Source: CAD feature listing. Evaluate the final solid. Frame: model axes, mm. Give positions to 0.01 mm unless a question says otherwise; leave off trailing zeros. Order: outer loops, then holes, each group sorted by start corner. A loop starts at its lowest first (then second) coordinate and runs counter-clockwise, first axis right, second up. Notation, with made-up numbers: (42, 19.5) - (46, 19.5) arc R21 ccw to (46, 34.5) - close; hole circle Ø6 at (59, 34.25). An arc over 180 degrees is marked (long way). Answer as CSV lines item,"result".
```python
from build123d import *

# Parameters (mm, degrees)
F0_R     = 12.7
F0_R_2   = 10.210562
F1_DEPTH = 1706.88
F2_R     = 6.35
F3_DEPTH = 25.4


with BuildPart() as f1:
    # F0 (on Right) → F1 (new body)
    with BuildSketch(Plane.YZ):
        Circle(F0_R)
        Circle(F0_R_2, mode=Mode.SUBTRACT)
    extrude(amount=F1_DEPTH)

    # F2 (on Top) → F3 (cut)
    with BuildSketch(Plane.XY):
        with Locations((341.376, 0)):
            Circle(F2_R)
        with Locations((682.752, 0)):
            Circle(F2_R)
        with Locations((1024.128, 0)):
            Circle(F2_R)
        with Locations((1365.504, 0)):
            Circle(F2_R)
    extrude(amount=F3_DEPTH, mode=Mode.SUBTRACT)


solid = f1.part
```
(1) Cut plane A-A (z = 0). Return loops of the section in (x, y), then the cut area to 3 significant figures.
Completed:
outline,"(0, -12.7) - (1706.88, -12.7) - (1706.88, -10.21) - (0, -10.21) - close; (0, 10.21) - (1706.88, 10.21) - (1706.88, 12.7) - (0, 12.7) - close"
area,"8,500 mm²"
(2) Cut plane B-B (y = 0). Return loops of the section in (x, z), then the cut area to 3 significant figures.
Completed:
outline,"(0, -12.7) - (1706.88, -12.7) - (1706.88, -10.21) - (0, -10.21) - close; (0, 10.21) - (335.03, 10.21) - (335.03, 12.7) - (0, 12.7) - close; (347.73, 10.21) - (676.4, 10.21) - (676.4, 12.7) - (347.73, 12.7) - close; (689.1, 10.21) - (1017.78, 10.21) - (1017.78, 12.7) - (689.1, 12.7) - close; (1030.48, 10.21) - (1359.15, 10.21) - (1359.15, 12.7) - (1030.48, 12.7) - close; (1371.85, 10.21) - (1706.88, 10.21) - (1706.88, 12.7) - (1371.85, 12.7) - close"
area,"8,370 mm²"
(3) Ray query, line 1 (X direction, y = 0, z = 11); line 2 (Z direction, x = 464.5, y = 7.75); line 3 (X direction, y = 2.5, z = 11). Return the intervals inside material, ascending. Write a range as from..to.
Completed:
line 1,"0..335.03, 347.73..676.4, 689.1..1017.78, 1030.48..1359.15, 1371.85..1706.88"
line 2,"-10.06..-6.65, 6.65..10.06"
line 3,"0..335.54, 347.21..676.91, 688.59..1018.29, 1029.97..1359.67, 1371.34..1706.88"
(4) Cut plane C-C (x = 1233). Return loops of the section in (y, z).
Completed:
outline,"circle Ø25.4 at (0, 0); hole circle Ø20.42 at (0, 0)"
(5) Contact query for flat-ended pins moving along their axis: pin 1 (2 mm diameter, centred on y = 6, z = -6.5, fed in from -X); pin 2 (8 mm diameter, centred on x = 433.5, y = -7, fed in from -Z); pin 3 (6 mm diameter, centred on x = 750.5, z = -5, fed in from +Y); pin 4 (5 mm diameter, centred on x = 590.5, y = 9.5, fed in from +Z). Output: stop coordinate, or through.
Completed:
pin 1,"through"
pin 2,"z = -12.34"
pin 3,"y = 12.54"
pin 4,"z = 10.6"
